```python
from build123d import *

# Parameters (mm, degrees)
F0_R     = 149.8
F0_R_2   = 99.8
F1_DEPTH = 70
F0_R_3   = 70
F2_DEPTH = 105
F6_DEPTH = 78.4
F8_D     = 10.5
F8_DEPTH = 149.801
F9_R     = 0.8


with BuildPart() as f1:
    # F0 (on Top) → F1 (new body)
    with BuildSketch(Plane.XY):
        Circle(F0_R)
        Circle(F0_R_2, mode=Mode.SUBTRACT)
    extrude(amount=F1_DEPTH)

    # F0 (on Top) → F2 (join)
    with BuildSketch(Plane.XY):
        Circle(F0_R_2)
        Circle(F0_R_3, mode=Mode.SUBTRACT)
    extrude(amount=F2_DEPTH)

    # F4: sweep along a path in F4_path
    with BuildLine(Plane(origin=(149.8, 0, 70), x_dir=(0, -1, 0), z_dir=(0, 0, -1))) as f4_path:
        CenterArc((0, 149.8), 149.8, 0, 360)
    # F3 (on Right) → F4 (sweep, cut)
    with BuildSketch(Plane.YZ):
        Polygon((-142.5000025749, 7.0000045449), (-149.8000025749, 7.0000045449), (-149.8000025749, 5.0000045449), align=None)
        Polygon((-142.5000025749, 63.0000045449), (-149.8000025749, 65.0000045449), (-149.8000025749, 7.0000045449), (-142.5000025749, 7.0000045449), align=None)
    sweep(path=f4_path.line, mode=Mode.SUBTRACT)

    # F5 (on Front) → F6 (cut)
    with BuildSketch(Plane.XZ):
        Polygon((-18, -125), (0, 0), (-18, 125), align=None)
        Polygon((0, -125), (18, -125), (0, 0), (-18, -125), align=None)
        Polygon((0, 0), (18, -125), (18, 125), align=None)
        Polygon((0, 0), (18, 125), (-18, 125), align=None)
    extrude(amount=-F6_DEPTH, mode=Mode.SUBTRACT)

    # F8 (through all, one way)
    with BuildSketch(Plane(origin=(0, 0, 0), x_dir=(0, 1, 0), z_dir=(-1, 0, 0))):
        with Locations((0, -85)):
            Circle(F8_D / 2)
    extrude(amount=-F8_DEPTH, mode=Mode.SUBTRACT)

    # F9
    f9_edges = [f1.edges().sort_by_distance(p)[0] for p in [
        (18, 78.4, 52.5),
        (-18, 78.4, 52.5),
    ]]
    fillet(f9_edges, radius=F9_R)


solid = f1.part
```
Model file for the job. Use its own axes, mm. A direction names the side the tool comes from. Coordinates: 2 decimals unless noted, no trailing zeros. Loops run counter-clockwise (first coordinate to the right, second up) from the corner with the lowest first, then second, coordinate; pieces in that order, holes last. Notation, with made-up numbers: (77, -37) - (86, -37) arc R14 cw to (86, -11) - close; hole circle Ø2 at (-34, -28.75). An arc over 180 degrees is marked (long way). Answer as a JSON object with one key per item and string values. Group by question number.
(1) Cut at D-D (z = 95). Give the cut face in (x, y).
(2) Probe line 1 along X through (y, z) = (0, 35); line 2 along Z through (x, y) = (81, 0); line 3 along Y through (x, z) = (10, 57). List the from-to ranges inside material, lowest first.
(3) Two-plate mould, pull along Z, no slides. Class faces 1 (the face through (21, 68, 105)), 2 (the face through (86.71, 113.08, 35.39)), 3 (the face through (0, 78.4, 53)): released by +Z, released by -Z, zero draft, split by the parting line, or undercut.
(4) Cut at A-A (x = 0). Give the cut face in (y, z), then the cut area to 3 significant figures.
(5) Cut at B-B (y = 0). Give the cut face in (x, z), then the cut area to 3 significant figures.
(6) Flat gauge pins, fed straight in: pin 1 (10 mm diameter, centred on x = -110.5, z = 56, fed in from -Y); pin 2 (17 mm diameter, centred on x = 3, z = 72, fed in from -Y); pin 3 (5 mm diameter, centred on x = -102.5, y = -14.5, fed in from +Z); pin 4 (13.5 mm diameter, centred on y = 0, z = 85, fed in from -X). Where does each tip first touch, or does it go through?
(7) Cut at C-C (z = 48). Give the cut face in (x, y).
(8) Tool access for faces 4 (the face through (64, -31, 0)), 5 (the face through (84.59, 2.82, 80.57)), 6 (the face through (18, 73, 52)), 7 (the face through (126.74, -65.92, 6.9)), 8 (the face through (31, -98, 70)): list every direction of +Z, -Z, +X, -X, +Y, -Y with a clear straight run to the whole face (end or side of a thin tool).
Geometry says:
{
 "1": {"outline": "circle Ø199.6 at (0, 0); hole (-18, 67.65) arc R70 ccw (long way) to (18, 67.65) - (18, 77.6) arc R0.8 ccw to (17.2, 78.4) - (-17.2, 78.4) arc R0.8 ccw to (-18, 77.6) - close"},
 "2": {"line 1": "x = -142.5 to -70, 70 to 142.5", "line 2": "z = 0 to 79.75, 90.25 to 105", "line 3": "y = -142.15 to -69.28, 78.4 to 142.15"},
 "3": {"face 1": "released by +Z", "face 2": "undercut", "face 3": "zero draft"},
 "4": {"outline": "(-149.8, 0) - (-70, 0) - (-70, 105) - (-99.8, 105) - (-99.8, 70) - (-149.8, 70) - (-149.8, 65) - (-142.5, 63) - (-142.5, 7) - (-149.8, 5) - close; (78.4, 0) - (149.8, 0) - (149.8, 5) - (142.5, 7) - (142.5, 63) - (149.8, 65) - (149.8, 70) - (99.8, 70) - (99.8, 105) - (78.4, 105) - close", "area": "11,500 mm^2"},
 "5": {"outline": "(-149.8, 0) - (-70, 0) - (-70, 105) - (-99.8, 105) - (-99.8, 70) - (-149.8, 70) - (-149.8, 65) - (-142.5, 63) - (-142.5, 7) - (-149.8, 5) - close; (70, 0) - (149.8, 0) - (149.8, 5) - (142.5, 7) - (142.5, 63) - (149.8, 65) - (149.8, 70) - (99.8, 70) - (99.8, 79.75) - (70, 79.75) - close; (70, 90.25) - (99.8, 90.25) - (99.8, 105) - (70, 105) - close", "area": "12,100 mm^2"},
 "6": {"pin 1": "stops at y = -95.79", "pin 2": "stops at y = -149.8", "pin 3": "stops at z = 70", "pin 4": "stops at x = -99.8"},
 "7": {"outline": "circle Ø285 at (0, 0); hole (-18, 67.65) arc R70 ccw (long way) to (18, 67.65) - (18, 77.6) arc R0.8 ccw to (17.2, 78.4) - (-17.2, 78.4) arc R0.8 ccw to (-18, 77.6) - close"},
 "8": {"face 4": "-Z, +X, -X, +Y, -Y", "face 5": "+X", "face 6": "+Z, -Z", "face 7": "none", "face 8": "+Z"}
}
